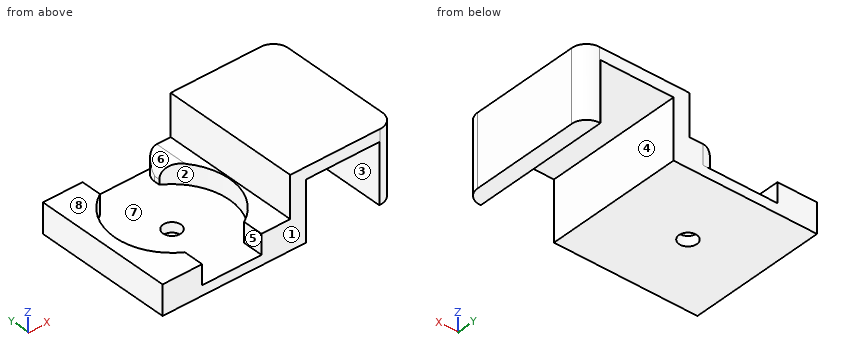
from build123d import *

# Parameters (mm, degrees)
PAD_DEPTH       = 7
SKETCH006_W     = 14
SKETCH006_H     = 14
PAD002_DEPTH    = 3
POCKET004_DEPTH = 2
SKETCH008_R     = 0.9
POCKET005_DEPTH = 1.001
FILLET_R        = 1.5


with BuildPart() as clamp_unit:
    # Sketch → Pad (new body, symmetric)
    with BuildSketch(Plane.XZ):
        Polygon((-3.7, 7.2), (5.3, 7.2), (5.3, 0), (3.7, 0), (3.7, 6), (-3.7, 6), (-3.7, 0), (-5.3, 0), (-5.3, 7.2), align=None)
    extrude(amount=PAD_DEPTH, both=True)


with BuildPart() as clone006:
    # Sketch006 → Pad002 (new body)
    with BuildSketch(Plane.XY):
        Rectangle(SKETCH006_W, SKETCH006_H)
    extrude(amount=PAD002_DEPTH)

    # Sketch007 → Pocket004 (cut)
    with BuildSketch(Plane.XY.offset(3)):
        with BuildLine():
            Line((-3, 7), (-3, 4.963869))
            ThreePointArc((-3, 4.963869), (-5.8, 0), (-3, -4.963869))
            Line((-3, -7), (-3, -4.963869))
            Line((3, -7), (-3, -7))
            Line((3, -4.963869), (3, -7))
            ThreePointArc((3, -4.963869), (5.8, 0), (3, 4.963869))
            Line((3, 7), (3, 4.963869))
            Line((-3, 7), (3, 7))
        make_face()
    extrude(amount=-POCKET004_DEPTH, mode=Mode.SUBTRACT)

    # Sketch008 → Pocket005 (cut, through all)
    with BuildSketch(Plane.XY.offset(1)):
        Circle(SKETCH008_R)
    extrude(amount=-POCKET005_DEPTH, mode=Mode.SUBTRACT)


with BuildPart() as clone006_1:
    # Clone placement: moved
    add(clone006.part.moved(Location((-11.2, 0, 0))))

    # Fusion: union clamp-unit
    add(clamp_unit.part)

    # Fillet
    fillet_edges = [clone006_1.edges().sort_by_distance(p)[0] for p in [
        (-8.2, 7, 2),
        (-8.2, 5.981935, 3),
        (5.3, 7, 3.6),
        (5.3, -7, 3.6),
    ]]
    fillet(fillet_edges, radius=FILLET_R)


with BuildPart() as clone006_2:
    # Clone006 placement: moved
    add(clone006_1.part.moved(Location((0, 30, 0))))


solid = clone006_2.part
Model file for the job. Use its own axes, mm. Face numbers are marked on the shaded views. A direction names the side the tool comes from. Coordinates: 2 decimals unless noted, no trailing zeros. Loops run counter-clockwise (first coordinate to the right, second up) from the corner with the lowest first, then second, coordinate; pieces in that order, holes last. Notation, with made-up numbers: (24, 6) -> (58, 6) arc R21 ccw to (58, 27) -> close; hole circle Ø2 at (37, 20). An arc over 180 degrees is marked (long way). Use one line per item in the form item = value. Start each with the question number.
(1) Cut at B-B on x = -11.2. Give the cut face in (y, z), and give its area (3 significant figures).
(2) Flat gauge pins, fed straight in: pin 1 (2 mm diameter, centred on x = -17, y = 33, fed in from +Z); pin 2 (0.6 mm diameter, centred on y = 24, z = 2.5, fed in from +X); pin 3 (2 mm diameter, centred on x = -0.5, y = 29, fed in from -Z). Where does each tip first touch, or does it go through?
(3) Cut at C-C on z = 2.25. Give the cut face in (x, y).
(4) Probe probe 1 along X at (y, z) = (24.75, 1.25); probe 2 along Y at (x, z) = (-11.2, 0.5); probe 3 along X at (y, z) = (33.75, 5.5). List the from-to ranges inside material, lowest first. Write a range as from..to.
(5) Tool access for the marked faces 4, 5, 6, 7 and 8: list every direction of +Z, -Z, +X, -X, +Y, -Y with a clear straight run to the whole face (end or side of a thin tool).
(6) Cut at A-A on y = 30. Give the cut face in (x, z).
(7) Cut at D-D on y = 36. Give the cut face in (x, z), and give its area (3 significant figures).
(8) Pull direction Y, two halves, no side cores. Call the marked faces 1, 2 and 3: pulls with the +Y half, pulls with the -Y half, needs draft (parallel to the pull), parting line crosses it, or undercut.
Values:
q1.outline = (23, 0) -> (29.1, 0) -> (29.1, 1) -> (23, 1) -> close; (30.9, 0) -> (37, 0) -> (37, 1) -> (30.9, 1) -> close
q1.area = 12.2 mm2
q2.pin_1 = 3
q2.pin_2 = 5.29
q2.pin_3 = 6
q3.outline = (-18.2, 23) -> (-14.2, 23) -> (-14.2, 25.04) arc R5.8 cw to (-14.2, 34.96) -> (-14.2, 37) -> (-18.2, 37) -> close; (-8.2, 23) -> (-3.7, 23) -> (-3.7, 37) -> (-6.7, 37) arc R1.5 ccw to (-8, 36.25) -> (-8, 34.84) arc R5.8 cw to (-8.2, 25.04) -> close; (3.7, 23) -> (3.8, 23) arc R1.5 ccw to (5.3, 24.5) -> (5.3, 35.5) arc R1.5 ccw to (3.8, 37) -> (3.7, 37) -> close
q4.probe_1 = -18.2..-14.2, -8.2..-3.7, 3.7..5.3
q4.probe_2 = 23..29.1, 30.9..37
q4.probe_3 = -5.3..-3.7, 3.7..5.3
q5.face_4 = -Z, +Y, -Y
q5.face_5 = +Z, +Y, -Y
q5.face_6 = +Z, +Y
q5.face_7 = +Z
q5.face_8 = +Z, -X, +Y, -Y
q6.outline = (-18.2, 0) -> (-12.1, 0) -> (-12.1, 1) -> (-17, 1) -> (-17, 3) -> (-18.2, 3) -> close; (-10.3, 0) -> (-3.7, 0) -> (-3.7, 6) -> (3.7, 6) -> (3.7, 0) -> (5.3, 0) -> (5.3, 7.2) -> (-5.3, 7.2) -> (-5.3, 3) -> (-5.4, 3) -> (-5.4, 1) -> (-10.3, 1) -> close
q7.outline = (-18.2, 0) -> (-3.7, 0) -> (-3.7, 6) -> (3.7, 6) -> (3.7, 0) -> (5.21, 0) -> (5.21, 7.2) -> (-5.3, 7.2) -> (-5.3, 3) -> (-6.7, 3) arc R1.5 ccw to (-8.11, 2) -> (-8.11, 1) -> (-14.2, 1) -> (-14.2, 3) -> (-18.2, 3) -> close
q7.area = 57.4 mm2
q8.face_1 = pulls with the -Y half
q8.face_2 = undercut
q8.face_3 = needs draft
